Build history of the part. All positions in model axes, mm. Face numbers are marked on the shaded views. A direction names the side the tool comes from. Round coordinates to 2 decimals unless told otherwise and drop trailing zeros. Write each loop counter-clockwise with the first axis right and the second up, starting at its lowest first coordinate (ties: lowest second). Pieces come first, ordered by that corner, then holes. Notation, with made-up numbers: (-29, 86.25) -> (3, 86.25) arc R30 ccw to (3, 113.25) -> close; hole circle Ø1 at (40.5, 71.25). An arc over 180 degrees is marked (long way). Answer in a Markdown table with one row per item.
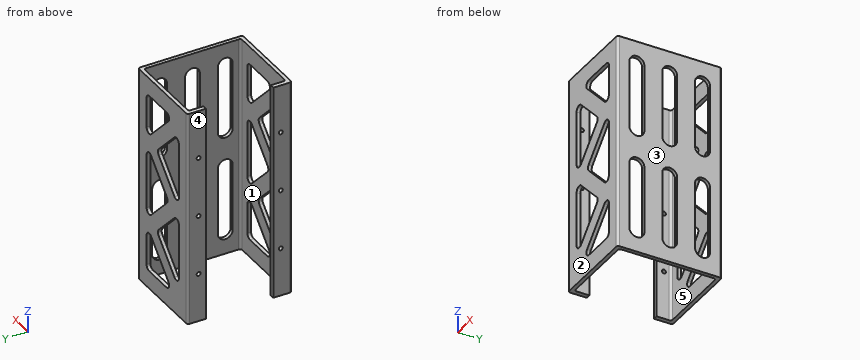
```python
from build123d import *

# Parameters (mm, degrees)
EXTRUDE_1_DEPTH     = 145
SKETCH_2_R          = 1.35
CUT_EXTRUDE_1_DEPTH = 3
CUT_EXTRUDE_2_DEPTH = 2.5
CUT_EXTRUDE_3_DEPTH = 70
FILLET_1_R          = 3
FILLET_2_R          = 1.5


with BuildPart() as part:
    # 草图1 → 凸台-拉伸1 (new body)
    with BuildSketch(Plane.XY):
        Polygon((0, 57.5), (0, 70), (57.5, 70), (57.5, 0), (0, 0), (0, 12.5), (3, 12.5), (3, 2.5), (55, 2.5), (55, 67.5), (3, 67.5), (3, 57.5), align=None)
    extrude(amount=-EXTRUDE_1_DEPTH)

    # 草图2 → 切除-拉伸1 (cut)
    with BuildSketch(Plane.ZY):
        with Locations((-112.5, 62.5)):
            Circle(SKETCH_2_R)
        with Locations((-72.5, 62.5)):
            Circle(SKETCH_2_R)
        with Locations((-32.5, 62.5)):
            Circle(SKETCH_2_R)
        with Locations((-32.5, 7.5)):
            Circle(SKETCH_2_R)
        with Locations((-72.5, 7.5)):
            Circle(SKETCH_2_R)
        with Locations((-112.5, 7.5)):
            Circle(SKETCH_2_R)
    extrude(amount=-CUT_EXTRUDE_1_DEPTH, mode=Mode.SUBTRACT)

    # 草图3 → 切除-拉伸2 (cut)
    with BuildSketch(Plane.ZY.offset(-55)):
        with BuildLine():
            Line((-130, 62), (-85, 62))
            ThreePointArc((-85, 62), (-80, 57), (-85, 52))
            Line((-85, 52), (-130, 52))
            ThreePointArc((-130, 52), (-135, 57), (-130, 62))
        make_face()
        with BuildLine():
            Line((-130, 40), (-85, 40))
            ThreePointArc((-85, 40), (-80, 35), (-85, 30))
            Line((-85, 30), (-130, 30))
            ThreePointArc((-130, 30), (-135, 35), (-130, 40))
        make_face()
        with BuildLine():
            Line((-130, 18), (-85, 18))
            ThreePointArc((-85, 18), (-80, 13), (-85, 8))
            Line((-85, 8), (-130, 8))
            ThreePointArc((-130, 8), (-135, 13), (-130, 18))
        make_face()
        with BuildLine():
            Line((-60, 62), (-15, 62))
            ThreePointArc((-15, 62), (-10, 57), (-15, 52))
            Line((-15, 52), (-60, 52))
            ThreePointArc((-60, 52), (-65, 57), (-60, 62))
        make_face()
        with BuildLine():
            Line((-60, 40), (-15, 40))
            ThreePointArc((-15, 40), (-10, 35), (-15, 30))
            Line((-15, 30), (-60, 30))
            ThreePointArc((-60, 30), (-65, 35), (-60, 40))
        make_face()
        with BuildLine():
            Line((-60, 18), (-15, 18))
            ThreePointArc((-15, 18), (-10, 13), (-15, 8))
            Line((-15, 8), (-60, 8))
            ThreePointArc((-60, 8), (-65, 13), (-60, 18))
        make_face()
    extrude(amount=-CUT_EXTRUDE_2_DEPTH, mode=Mode.SUBTRACT)

    # 草图4 → 切除-拉伸3 (cut)
    with BuildSketch(Plane(origin=(0, 70, 0), x_dir=(1, 0, 0), z_dir=(0, 1, 0))):
        Polygon((47.5, 98.095598855), (21.904401145, 72.5), (47.5, 46.904401145), align=None)
        Polygon((17.071067812, 133), (47.5, 102.571067812), (47.5, 133), align=None)
        Polygon((10, 125.928932188), (35.595598855, 100.333333333), (10, 74.737734479), align=None)
        Polygon((10, 70.262265521), (35.595598855, 44.666666667), (10, 19.071067812), align=None)
        Polygon((17.071067812, 12), (47.5, 42.428932188), (47.5, 12), align=None)
    extrude(amount=-CUT_EXTRUDE_3_DEPTH, mode=Mode.SUBTRACT)

    # 圆角1
    fillet_1_edges = [part.edges().sort_by_distance(p)[0] for p in [
        (17.071067812, 1.25, -133),
        (47.5, 1.25, -133),
        (47.5, 1.25, -102.571067812),
        (17.071067812, 68.75, -133),
        (47.5, 68.75, -133),
        (47.5, 68.75, -102.571067812),
        (47.5, 1.25, -98.095598855),
        (47.5, 1.25, -46.904401145),
        (21.904401145, 1.25, -72.5),
        (47.5, 68.75, -98.095598855),
        (47.5, 68.75, -46.904401145),
        (21.904401145, 68.75, -72.5),
        (10, 1.25, -74.737734479),
        (10, 1.25, -125.928932188),
        (35.595598855, 1.25, -100.333333333),
        (10, 68.75, -74.737734479),
        (10, 68.75, -125.928932188),
        (35.595598855, 68.75, -100.333333333),
        (10, 1.25, -19.071067812),
        (10, 1.25, -70.262265521),
        (35.595598855, 1.25, -44.666666667),
        (10, 68.75, -19.071067812),
        (10, 68.75, -70.262265521),
        (35.595598855, 68.75, -44.666666667),
        (47.5, 1.25, -12),
        (17.071067812, 1.25, -12),
        (47.5, 1.25, -42.428932188),
        (47.5, 68.75, -12),
        (17.071067812, 68.75, -12),
        (47.5, 68.75, -42.428932188),
    ]]
    fillet(fillet_1_edges, radius=FILLET_1_R)

    # 圆角2
    fillet_2_edges = [part.edges().sort_by_distance(p)[0] for p in [
        (0, 70, -72.5),
        (57.5, 70, -72.5),
        (57.5, 0, -72.5),
        (0, 0, -72.5),
        (3, 2.5, -72.5),
        (55, 2.5, -72.5),
        (55, 67.5, -72.5),
        (3, 67.5, -72.5),
    ]]
    fillet(fillet_2_edges, radius=FILLET_2_R)


solid = part.part
```
Q1. Saw through at B-B on x = 19.5. Write the cut outline in (y, z).
A:
| item | result |
|---|---|
| outline | (0, -145) -> (2.5, -145) -> (2.5, -116.43) -> (0, -116.43) -> close; (0, -84.24) -> (2.5, -84.24) -> (2.5, -60.76) -> (0, -60.76) -> close; (0, -28.57) -> (2.5, -28.57) -> (2.5, 0) -> (0, 0) -> close; (67.5, -145) -> (70, -145) -> (70, -116.43) -> (67.5, -116.43) -> close; (67.5, -84.24) -> (70, -84.24) -> (70, -60.76) -> (67.5, -60.76) -> close; (67.5, -28.57) -> (70, -28.57) -> (70, 0) -> (67.5, 0) -> close |
Q2. Which spindle directions (+Z, -Z, +X, -X, +Y, -Y) get a long thin tool onto all of the face, cutting with end or side? Do the marked faces 4 and 5. Say none if no direction does.
A:
| item | result |
|---|---|
| face 4 | +Z, -Z, -X, +Y, -Y |
| face 5 | +Z, -Z |
Q3. Saw through at C-C on y = 16. Write the cut outline in (x, z).
A:
| item | result |
|---|---|
| outline | (55, -145) -> (57.5, -145) -> (57.5, -134) -> (55, -134) -> close; (55, -81) -> (57.5, -81) -> (57.5, -64) -> (55, -64) -> close; (55, -11) -> (57.5, -11) -> (57.5, 0) -> (55, 0) -> close |
Q4. Drop flat-ended pins along their axis: P1, Ø4, axis at y = 33.5, z = -46, coming from the +X side; P2, Ø7, axis at y = 8.5, z = -94.5, coming from the +X side; P3, Ø1.2, axis at x = 57, z = -110, coming from the -Y side; P4, Ø10, axis at y = 39.5, z = -94.5, coming from the -X side. Give the stop position or say it passes through.
A:
| item | result |
|---|---|
| P1 | through |
| P2 | x = 57.5 |
| P3 | y = 0.05 |
| P4 | x = 55 |
Q5. Two-plate mould, pull along Y, no slides. Class the marked faces 1, 2 and 3: released by +Y, released by -Y, zero draft, split by the parting line, or undercut.
A:
| item | result |
|---|---|
| face 1 | undercut |
| face 2 | released by -Y |
| face 3 | zero draft |
Q6. Saw through at D-D on z = -104.5. State how many separate pieces and enclosed holes the cut face has, plus the area to 3 significant figures.
A:
| item | result |
|---|---|
| separate pieces | 6 |
| enclosed holes | 0 |
| area | 328 mm² |
Q7. Wall check: line 1 (Y direction, x = 1.85, z = -112.5); line 2 (Y direction, x = 34, z = -40); line 3 (X direction, y = 62.5, z = -18). Give the ranges that are in metal, low to high. Write a range as [from, to].
A:
| item | result |
|---|---|
| line 1 | [0, 6.15], [8.85, 12.5], [57.5, 61.15], [63.85, 70] |
| line 2 | [0, 2.5], [67.5, 70] |
| line 3 | [0, 3], [55, 57.5] |
Q8. Saw through at A-A on y = 35. Write the cut outline in (x, z), plus the area to 3 significant figures.
A:
| item | result |
|---|---|
| outline | (55, -145) -> (57.5, -145) -> (57.5, -135) -> (55, -135) -> close; (55, -80) -> (57.5, -80) -> (57.5, -65) -> (55, -65) -> close; (55, -10) -> (57.5, -10) -> (57.5, 0) -> (55, 0) -> close |
| area | 87.5 mm² |
